Read the model definition and answer for the solid it produces. Units are mm, in the model's axes. Round coordinates to 2 decimals unless told otherwise and drop trailing zeros. Order: outer loops, then holes, each group sorted by start corner. A loop starts at its lowest first (then second) coordinate and runs counter-clockwise, first axis right, second up. Notation, with made-up numbers: (-30.5, 28) - (-16.5, 28) arc R9 ccw to (-16.5, 35) - close; hole circle Ø10 at (14, -3.5). An arc over 180 degrees is marked (long way). Answer as a JSON object with one key per item and string values. Group by question number.
Q1. A cutting plane is placed at C-C on y = 7.25. Count the separate pieces of the cut face and the enclosed holes in it, and give its area (3 significant figures).
Q2. A cutting plane is placed at B-B on z = -5.75. Determine the outline of the cut face in (x, y).
Q3. Given pin 1 Ø7 at (x, z) = (-5, -2) entering from +Y; pin 2 Ø5.5 at (y, z) = (21.33, -8.62) entering from +X; pin 3 Ø5 at (y, z) = (12, -1) entering from -X, each flat-ended and moving along its own axis, determine where each tip first touches the part or whether it passes through.
Q4. Consider line 1 (Z direction, x = -9, y = 1.5); line 2 (Y direction, x = 15, z = 7.5); line 3 (Y direction, x = -7, z = 7.5). Determine where each line is inside the solid, lowest interval first.
Q5. The mould has two halves that part along Y. Classify faces 1 (the cylindrical face through (14.453, 21.838, 10.246)), 2 (the flat face through (5.7, 4.8, -12)), 3 (the flat face through (14, 24, 0)), 4 (the flat face through (0, 0, 0)): pulls with the +Y half, pulls with the -Y half, needs draft (parallel to the pull), parting line crosses it, or undercut.
Q6. A cutting plane is placed at A-A on x = -9. Determine the outline of the cut face in (y, z) (3 decimals), and give its area (3 significant figures).
```python
from build123d import *

# Parameters (mm, degrees)
SKETCH1_W                      = 24
SKETCH1_H                      = 24
BOSS_EXTRUDE1_DEPTH            = 5
BOSS_EXTRUDE2_START            = 12
SKETCH2_W                      = 24
SKETCH2_H                      = 24
BOSS_EXTRUDE2_DEPTH            = 5
FILLET3_R                      = 5
M3_CLEARANCE_HOLE1_D           = 3.4
M3_CLEARANCE_HOLE1_CSINK_D     = 3.45
M3_CLEARANCE_HOLE1_CSINK_ANGLE = 90
M3_CLEARANCE_HOLE2_D           = 3.4
M3_CLEARANCE_HOLE2_CSINK_D     = 3.45
M3_CLEARANCE_HOLE2_CSINK_ANGLE = 90


with BuildPart() as part:
    # Sketch1 → Boss-Extrude1 (new body)
    with BuildSketch(Plane(origin=(0, 0, 0), x_dir=(1, 0, 0), z_dir=(0, 1, 0))):
        Rectangle(SKETCH1_W, SKETCH1_H)
    extrude(amount=BOSS_EXTRUDE1_DEPTH)

    # Sketch2 → Boss-Extrude2 (add)
    with BuildSketch(Plane(origin=(0, 0, 0), x_dir=(0, 0, -1), z_dir=(1, 0, 0)).offset(BOSS_EXTRUDE2_START)):
        with Locations((0, 12)):
            Rectangle(SKETCH2_W, SKETCH2_H)
    extrude(amount=BOSS_EXTRUDE2_DEPTH)

    # Fillet3
    fillet3_edges = [part.edges().sort_by_distance(p)[0] for p in [
        (17, 0, 0),
    ]]
    fillet(fillet3_edges, radius=FILLET3_R)

    # M3 Clearance Hole1 (through all)
    with Locations(Plane(origin=(17, 0, 0), x_dir=(0, 0, -1), z_dir=(1, 0, 0))):
        with Locations((-8.624504069, 21.327732388), (8.624504069, 21.327732388), (8.624504069, 7.672267612), (-8.624504069, 7.672267612)):
            CounterSinkHole(M3_CLEARANCE_HOLE1_D / 2, M3_CLEARANCE_HOLE1_CSINK_D / 2, counter_sink_angle=M3_CLEARANCE_HOLE1_CSINK_ANGLE)

    # M3 Clearance Hole2 (through all)
    with Locations(Plane(origin=(0, 5, 0), x_dir=(1, 0, 0), z_dir=(0, 1, 0))):
        with Locations((-9, -9), (-9, 9.203654699), (9.203654699, 9.203654699), (9.203654699, -9)):
            CounterSinkHole(M3_CLEARANCE_HOLE2_D / 2, M3_CLEARANCE_HOLE2_CSINK_D / 2, counter_sink_angle=M3_CLEARANCE_HOLE2_CSINK_ANGLE)


solid = part.part
```
Result set:
{
 "1": {"separate pieces": "3", "enclosed holes": "0", "area": "87.1 mm²"},
 "2": {"outline": "(-12, 0) - (12, 0) arc R5 ccw to (17, 5) - (17, 24) - (12, 24) - (12, 5) - (-12, 5) - close"},
 "3": {"pin 1": "stops at y = 5", "pin 2": "stops at x = 17", "pin 3": "stops at x = 12"},
 "4": {"line 1": "z = -12 to -10.9, -7.5 to 7.3, 10.7 to 12", "line 2": "y = 1 to 6.4, 8.95 to 20.05, 22.6 to 24", "line 3": "y = 0 to 5"},
 "5": {"face 1": "undercut", "face 2": "needs draft", "face 3": "pulls with the +Y half", "face 4": "pulls with the -Y half"},
 "6": {"outline": "(0, -12) - (5, -12) - (5, -10.929) - (4.975, -10.904) - (0, -10.904) - close; (0, -7.504) - (4.975, -7.504) - (5, -7.479) - (5, 7.275) - (4.975, 7.3) - (0, 7.3) - close; (0, 10.7) - (4.975, 10.7) - (5, 10.725) - (5, 12) - (0, 12) - close", "area": "86.0 mm²"}
}
